Design review of the part built by this model. Coordinates are the model's own, in mm. A direction names the side the tool comes from. Give positions to 0.01 mm unless a question says otherwise; leave off trailing zeros. Order: outer loops, then holes, each group sorted by start corner. A loop starts at its lowest first (then second) coordinate and runs counter-clockwise, first axis right, second up. Notation, with made-up numbers: (77.5, -0.5) -> (113.5, -0.5) arc R16 cw to (113.5, 10.5) -> close; hole circle Ø6 at (-8.5, 23.25). An arc over 180 degrees is marked (long way). Answer in a Markdown table with one row per item. Add a question column.
Solid Edge part; units mm, degrees
sketch "Sketch1" plane through (0, 0, 0) normal (0, 0, 1) x (1, 0, 0)
  line L0 (-78.7684, 102.3579) -> (-70.7684, 102.3579)
  line L1 (-70.7684, 102.3579) -> (-70.7684, 30.3579)
  line L2 (-70.7684, 30.3579) -> (38.2316, 30.3579)
  line L3 (38.2316, 30.3579) -> (38.2316, 102.3579)
  line L4 (38.2316, 102.3579) -> (46.2316, 102.3579)
  line L5 (46.2316, 102.3579) -> (46.2316, 22.3579)
  line L6 (46.2316, 22.3579) -> (-78.7684, 22.3579)
  line L7 (-78.7684, 22.3579) -> (-78.7684, 102.3579)
  dimension "D1" = 78.7684
extrude "Protrusion1" add sketch "Sketch1" along normal blind 150
sketch "Sketch2" plane through (-16.2684, 22.3579, 75) normal (0, -1, 0) x (1, 0, 0)
  circle A0 centre (0, -10) radius 5
extrude "Cutout1" cut sketch "Sketch2" against normal through all
sketch "Sketch3" plane through (-16.2684, 22.3579, 75) normal (0, -1, 0) x (1, 0, 0)
  circle A0 centre (0, -10) radius 12.5
extrude "ExtrudedCutout_2" cut sketch "Sketch3" against normal blind 1
hole "Hole_1" at (46.2316, 73.3579, 75) direction (-1, 0, 0) diameter 6.5 end up to next
hole "Hole1" at (46.2316, 73.3579, 15) direction (-1, 0, 0) diameter 6.5 end up to next
hole "Hole2" at (46.2316, 73.3579, 135) direction (-1, 0, 0) diameter 6.5 end up to next
properties material "Aluminum, 6061-T6"
1) Add section C-C, the plane x = -13.5. Write out the cut boundary in (y, z).
2) Machinability: for faces 1 (the face through (-25.48, 22.85, 73.45)), 2 (the face through (38.232, 66, 74)), 3 (the face through (42.29, 75.55, 77.4)), 4 (the face through (-13.58, 26.809, 69.216)), which of the approach directions +Z, -Z, +X, -X, +Y, -Y give a long, thin tool a straight path to every point of the face, cutting with its end or side? Answer none if there is none.
3) Mouldability with a two-part tool opening along X and no side actions: class faces 5 (the face through (-78.768, 62, 74)), 6 (the face through (-22, 23.358, 65)), 7 (the face through (42.29, 76.58, 15.42)) as +X half, -X half, draft (parallel to the pull), parting line (faces both ways), or undercut.
4) Add section B-B, the plane y = 89.5. Write out the cut boundary in (x, z).
5) Add section D-D, the plane z = 65. Write out the cut boundary in (x, y), and give its area (3 significant figures).
6) Clearance check with flat-ended pins moving along their axes: P1, Ø1.5, axis at x = -5.5, z = 121, coming from the +Y side; P2, Ø15, axis at x = -16.27, z = 65, coming from the -Y side. State where each tip first meets the part, or that it passes through.
7) Add section A-A, the plane z = 15. Write out the cut boundary in (x, y).
8) For L1, parallel to X at y = 35.5, z = 122; L2, parallel to Y at x = 41.75, z = 75; L3, parallel to Y at x = -58, z = 20, list the stretches that pass through material, from the lowest coordinate up.
Verdict:
| question | item | result |
|---|---|---|
| 1 | outline | (22.36, 0) -> (30.36, 0) -> (30.36, 60.84) -> (23.36, 60.84) -> (23.36, 52.81) -> (22.36, 52.81) -> close; (22.36, 77.19) -> (23.36, 77.19) -> (23.36, 69.16) -> (30.36, 69.16) -> (30.36, 150) -> (22.36, 150) -> close |
| 2 | face 1 | -Y |
| 2 | face 2 | +Z, -Z, +Y |
| 2 | face 3 | +X |
| 2 | face 4 | +Y, -Y |
| 3 | face 5 | -X half |
| 3 | face 6 | undercut |
| 3 | face 7 | draft |
| 4 | outline | (-78.77, 0) -> (-70.77, 0) -> (-70.77, 150) -> (-78.77, 150) -> close; (38.23, 0) -> (46.23, 0) -> (46.23, 150) -> (38.23, 150) -> close |
| 5 | outline | (-78.77, 22.36) -> (-28.77, 22.36) -> (-28.77, 23.36) -> (-21.27, 23.36) -> (-21.27, 30.36) -> (-70.77, 30.36) -> (-70.77, 102.36) -> (-78.77, 102.36) -> close; (-11.27, 23.36) -> (-3.77, 23.36) -> (-3.77, 22.36) -> (46.23, 22.36) -> (46.23, 102.36) -> (38.23, 102.36) -> (38.23, 30.36) -> (-11.27, 30.36) -> close |
| 5 | area | 2,060 mm2 |
| 6 | P1 | stops at y = 30.36 |
| 6 | P2 | stops at y = 23.36 |
| 7 | outline | (-78.77, 22.36) -> (46.23, 22.36) -> (46.23, 70.11) -> (38.23, 70.11) -> (38.23, 30.36) -> (-70.77, 30.36) -> (-70.77, 102.36) -> (-78.77, 102.36) -> close; (38.23, 76.61) -> (46.23, 76.61) -> (46.23, 102.36) -> (38.23, 102.36) -> close |
| 8 | L1 | x = -78.77 to -70.77, 38.23 to 46.23 |
| 8 | L2 | y = 22.36 to 70.11, 76.61 to 102.36 |
| 8 | L3 | y = 22.36 to 30.36 |
